Geometry: final body of the model. Coordinates: model frame, mm. Face numbers are marked on the shaded views. Give positions to 0.01 mm unless a question says otherwise; leave off trailing zeros. Loops run counter-clockwise (first coordinate to the right, second up) from the corner with the lowest first, then second, coordinate; pieces in that order, holes last.
Autodesk Inventor part; units mm, degrees
ref_plane "YZ Plane" through (0, 0, 0) normal (1, 0, 0) x (0, 1, 0)
ref_plane "XZ Plane" through (0, 0, 0) normal (0, 1, 0) x (-1, 0, 0)
ref_plane "XY Plane" through (0, 0, 0) normal (0, 0, 1) x (1, 0, 0)
sketch "Sketch1" plane through (0, 0, 0) normal (0, 0, 1) x (1, 0, 0)
  arc A0 (-22.5975, -105.4525) -> (-31.0052, -218.9372) centre (-30.2027, -161.9428) ccw
  arc A1 (419.3749, -225.2787) -> (423.8, -165.5499) centre (419.7973, -195.2817) ccw
  line L0 (-22.5975, -105.4525) -> (423.8, -165.5499)
  line L1 (-31.0052, -218.9372) -> (419.3749, -225.2787)
  arc A2 (-22.4265, -104.1818) -> (-31.0232, -220.2191) centre (-30.2027, -161.9428) ccw
  line L2 (-22.4265, -104.1818) -> (423.9711, -164.2793)
  arc A3 (419.3569, -226.5607) -> (423.9711, -164.2793) centre (419.7973, -195.2817) ccw
  line L3 (419.3569, -226.5607) -> (-31.0232, -220.2191)
  arc A4 (-27.7033, -103.7144) -> (-32.7021, -103.7144) centre (-30.2027, -103.6607) ccw
  point P0 (0, 0)
  dimension "d1" = 57
  dimension "d2" = 30
  dimension "d3" = 450
  dimension "d4" = 1.2821
  dimension "d7" = 5
extrude "Extrusion1" add sketch "Sketch1" along normal blind 31 contours L2 A3 L3 A2
sketch "Sketch2" plane through (0, 0, 0) normal (0, 0, -1) x (-1, 0, 0)
  point P0 (0, 0)
extrude "Extrusion3" [suppressed]
equation "\"d1\" = 0.5 * NagyKerekAtmero"
equation "\"d2\" = 0.5 * KisKerekAtmero"
equation "\"d5\" = SzíjSzélességA"
properties part number "Szij"
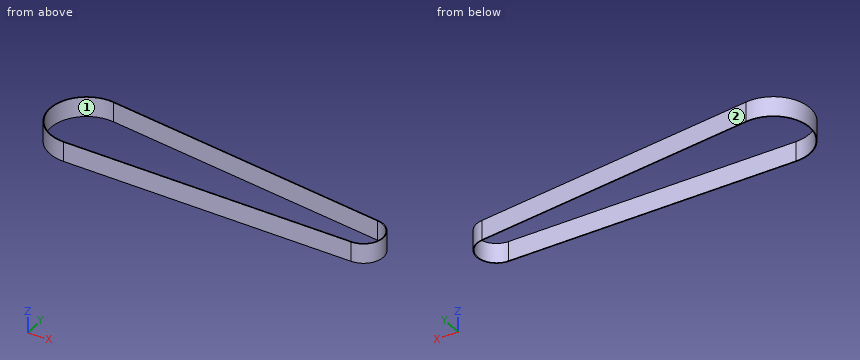
Item 1: Section query C-C on y = -175. Return loops of the section in (x, z).
Values follow:
outline: (-87, 0) - (-85.69, 0) - (-85.69, 31) - (-87, 31) - close; (441.9, 0) - (443.61, 0) - (443.61, 31) - (441.9, 31) - close
Item 2: Ray query, probe 1 along X at (y, z) = (-195.5, 2.5); probe 2 along Y at (x, z) = (101.5, 15); probe 3 along Y at (x, z) = (189.5, 22.5). Return the intervals inside material, ascending.
Values follow:
probe 1: x = -77.85 to -76.28, 449.8 to 451.08
probe 2: y = -222.09 to -220.8, -122.16 to -120.87
probe 3: y = -223.32 to -222.04, -134.01 to -132.71
Item 3: Section query A-A on z = 21. Return loops of the section in (x, y).
Values follow:
outline: (-31.02, -220.22) - (419.36, -226.56) arc R31.28 ccw to (423.97, -164.28) - (-22.43, -104.18) arc R58.28 ccw (long way) to start; hole (-31.01, -218.94) - (419.37, -225.28) arc R30 ccw to (423.8, -165.55) - (-22.6, -105.45) arc R57 ccw (long way) to start
Item 4: Draft query along X for the marked faces 1 and 2. Return one class per face: +X half, -X half, draft (parallel to the pull), parting line (faces both ways), or undercut.
Values follow:
face 1: undercut
face 2: +X half
Item 5: Pin query (flat end, axial travel): pin 1 (4 mm diameter, centred on y = -153.5, z = 14.5, fed in from -X); pin 2 (5 mm diameter, centred on x = 36.5, z = 26.5, fed in from +Y); pin 3 (12 mm diameter, centred on x = 387, y = -160.5, fed in from -Z); pin 4 (5 mm diameter, centred on y = -214, z = 23, fed in from -X). Return the tip coordinate at first contact, or that it passes through.
Values follow:
pin 1: stops at x = -88.13
pin 2: stops at y = -111.78
pin 3: stops at z = 0
pin 4: stops at x = -60.88
